Can you work these out from the model? Positions are in its coordinate system, mm. Face numbers are marked on the shaded views. A direction names the side the tool comes from. Round coordinates to 2 decimals unless told otherwise and drop trailing zeros. Write each loop counter-clockwise with the first axis right and the second up, starting at its lowest first coordinate (ties: lowest second). Pieces come first, ordered by that corner, then holes. Notation, with made-up numbers: (-17, 76) -> (32, 76) arc R14 ccw to (32, 80) -> close; hole circle Ø3 at (46, 10). An arc over 180 degrees is marked (long way). Write item = value, one per line. Start each with the question number.
1) If I drill on line 1 (Y direction, x = 154.5, z = 96); line 2 (X direction, y = 126, z = 8); line 3 (Y direction, x = 157.5, z = -145), over which ranges is the centre line in solid material (lowest first)?
2) For the marked faces 1 and 2, which set-ups out of +Z, -Z, +X, -X, +Y, -Y let a thin tool reach every point of the face, with its end or its side?
3) I'm going to push flat-ended pins straight in: pin 1 (24 mm diameter, centred on x = 241, y = 206, fed in from +Z); pin 2 (8 mm diameter, centred on y = 297.5, z = 144, fed in from +X); pin 3 (5.5 mm diameter, centred on x = -153, y = -194.5, fed in from +Z). Where does each tip first touch, or does it pass through?
4) Imagine slicing it at A-A, the plane y = 260.5. Please give me the cut outline in (x, z), then the cut area to 3 significant figures.
5) Imagine slicing it at C-C, the plane x = 54.5. Please give me the cut outline in (y, z).
6) Imagine slicing it at B-B, the plane z = -93.5. State how many separate pieces and enclosed holes the cut face has, then the cut area to 3 significant figures.
7) Imagine slicing it at D-D, the plane x = 182. Please give me the cut outline in (y, z).
8) Thinking about a two-plate mould opening in Y: for the marked faces 3, 4, 5 and 6, which applies, +Y half, -Y half, draft (parallel to the pull), parting line (faces both ways), or undercut?
from build123d import *

# Parameters (mm, degrees)
SKETCH1_W            = 450
SKETCH1_H            = 900
BOSS_EXTRUDE1_DEPTH  = 225
SKETCH2_W            = 390
SKETCH2_H            = 870
CUT_EXTRUDE1_DEPTH   = 420
SKETCH3_W            = 390
SKETCH3_H            = 390
BOSS_EXTRUDE2_DEPTH  = 30
LPATTERN1_COUNT      = 3
LPATTERN1_PITCH      = 155
SKETCH5_W            = 325
SKETCH5_H            = 350.459165748
SKETCH5_W_2          = 265
SKETCH5_H_2          = 290.459165748
BOSS_EXTRUDE4_DEPTH  = 390
SKETCH6_W            = 390
SKETCH6_H            = 125
BOSS_EXTRUDE5_DEPTH  = 10
LPATTERN2_COUNT      = 2
LPATTERN2_PITCH      = 155
LPATTERN2_COUNT_DIR2 = 2
LPATTERN2_PITCH_DIR2 = 320
CUT_EXTRUDE2_REACH   = 632.496
SKETCH10_R           = 2.5
LPATTERN3_COUNT      = 2
LPATTERN3_PITCH      = 155
LPATTERN3_COUNT_DIR2 = 2
LPATTERN3_PITCH_DIR2 = 320
SKETCH13_W           = 450
SKETCH13_H           = 30
BOSS_EXTRUDE6_DEPTH  = 30
CUT_EXTRUDE4_REACH   = 677
SKETCH12_R           = 2.5
CUT_EXTRUDE5_START   = -10
SKETCH17_R           = 2.5
CUT_EXTRUDE5_DEPTH   = 677.276969435
SKETCH18_W           = 53
SKETCH18_H           = 30
CUT_EXTRUDE6_DEPTH   = 676
SKETCH19_W           = 53
SKETCH19_H           = 30
CUT_EXTRUDE7_DEPTH   = 30
SKETCH20_R           = 2.5
CUT_EXTRUDE8_DEPTH   = 10


with BuildPart() as part:
    # Sketch1 → Boss-Extrude1 (new, symmetric)
    with BuildSketch(Plane(origin=(0, 0, 0), x_dir=(0, 0, -1), z_dir=(1, 0, 0))):
        Rectangle(SKETCH1_W, SKETCH1_H)
    extrude(amount=BOSS_EXTRUDE1_DEPTH, both=True)

    # Sketch2 → Cut-Extrude1 (cut)
    with BuildSketch(Plane.XY.offset(225)):
        with Locations((0, -15)):
            Rectangle(SKETCH2_W, SKETCH2_H)
    extrude(amount=-CUT_EXTRUDE1_DEPTH, mode=Mode.SUBTRACT)

    # Sketch3 → Boss-Extrude2 (add)
    with BuildSketch(Plane(origin=(0, 320, 0), x_dir=(1, 0, 0), z_dir=(0, 1, 0))):
        Rectangle(SKETCH3_W, SKETCH3_H)
    boss_extrude2 = extrude(amount=-BOSS_EXTRUDE2_DEPTH)

    # LPattern1: Boss-Extrude2 ×3
    with Locations(*[(0, -i * LPATTERN1_PITCH, 0) for i in range(1, LPATTERN1_COUNT)]):
        add(boss_extrude2)

    # Sketch5 → Boss-Extrude4 (add)
    with BuildSketch(Plane.XY.offset(-195)):
        with Locations((2.5, -274.770417126)):
            Rectangle(SKETCH5_W, SKETCH5_H)
        with Locations((2.5, -274.770417126)):
            Rectangle(SKETCH5_W_2, SKETCH5_H_2, mode=Mode.SUBTRACT)
    extrude(amount=BOSS_EXTRUDE4_DEPTH)

    # Sketch6 → Boss-Extrude5 (add)
    with BuildSketch(Plane(origin=(-165, 0, 0), x_dir=(0, 0, -1), z_dir=(1, 0, 0))):
        with Locations((0, 227.5)):
            Rectangle(SKETCH6_W, SKETCH6_H)
    boss_extrude5 = extrude(amount=BOSS_EXTRUDE5_DEPTH)

    # LPattern2: Boss-Extrude5 2 × 2
    with Locations(*[(j * LPATTERN2_PITCH_DIR2, -i * LPATTERN2_PITCH, 0) for i in range(LPATTERN2_COUNT) for j in range(LPATTERN2_COUNT_DIR2) if (i, j) != (0, 0)]):
        add(boss_extrude5)

    # Sketch10 → Cut-Extrude2 (cut, up to next)
    with BuildSketch(Plane(origin=(-155, 0, 0), x_dir=(0, 0, -1), z_dir=(1, 0, 0)), mode=Mode.PRIVATE) as cut_extrude2_sk1:
        with Locations((-165, 225)):
            Circle(SKETCH10_R)
    cut_extrude2_tool1 = extrude(cut_extrude2_sk1.sketch, amount=-CUT_EXTRUDE2_REACH, mode=Mode.PRIVATE) & part.part
    # Sketch10 → Cut-Extrude2 (cut, up to next)
    with BuildSketch(Plane(origin=(-155, 0, 0), x_dir=(0, 0, -1), z_dir=(1, 0, 0)), mode=Mode.PRIVATE) as cut_extrude2_sk2:
        with Locations((-145, 225)):
            Circle(SKETCH10_R)
    cut_extrude2_tool2 = extrude(cut_extrude2_sk2.sketch, amount=-CUT_EXTRUDE2_REACH, mode=Mode.PRIVATE) & part.part
    # Sketch10 → Cut-Extrude2 (cut, up to next)
    with BuildSketch(Plane(origin=(-155, 0, 0), x_dir=(0, 0, -1), z_dir=(1, 0, 0)), mode=Mode.PRIVATE) as cut_extrude2_sk3:
        with Locations(Location((145, 225, 0), (0, 0, 180))):
            Circle(SKETCH10_R)
    cut_extrude2_tool3 = extrude(cut_extrude2_sk3.sketch, amount=-CUT_EXTRUDE2_REACH, mode=Mode.PRIVATE) & part.part
    # Sketch10 → Cut-Extrude2 (cut, up to next)
    with BuildSketch(Plane(origin=(-155, 0, 0), x_dir=(0, 0, -1), z_dir=(1, 0, 0)), mode=Mode.PRIVATE) as cut_extrude2_sk4:
        with Locations(Location((165, 225, 0), (0, 0, 180))):
            Circle(SKETCH10_R)
    cut_extrude2_tool4 = extrude(cut_extrude2_sk4.sketch, amount=-CUT_EXTRUDE2_REACH, mode=Mode.PRIVATE) & part.part
    cut_extrude2_1 = cut_extrude2_tool1.solids().sort_by_distance((-155, 225, 165))[0]
    add(cut_extrude2_1, mode=Mode.SUBTRACT)
    cut_extrude2_2 = cut_extrude2_tool2.solids().sort_by_distance((-155, 225, 145))[0]
    add(cut_extrude2_2, mode=Mode.SUBTRACT)
    cut_extrude2_3 = cut_extrude2_tool3.solids().sort_by_distance((-155, 225, -145))[0]
    add(cut_extrude2_3, mode=Mode.SUBTRACT)
    cut_extrude2_4 = cut_extrude2_tool4.solids().sort_by_distance((-155, 225, -165))[0]
    add(cut_extrude2_4, mode=Mode.SUBTRACT)
    cut_extrude2 = cut_extrude2_1 + cut_extrude2_2 + cut_extrude2_3 + cut_extrude2_4  # Cut-Extrude2 as one shape, for the pattern or mirror that repeats it

    # LPattern3: Cut-Extrude2 2 × 2
    with Locations(*[(j * LPATTERN3_PITCH_DIR2, -i * LPATTERN3_PITCH, 0) for i in range(LPATTERN3_COUNT) for j in range(LPATTERN3_COUNT_DIR2) if (i, j) != (0, 0)]):
        add(cut_extrude2, mode=Mode.SUBTRACT)

    # Sketch13 → Boss-Extrude6 (add)
    with BuildSketch(Plane(origin=(225, 0, 0), x_dir=(0, 0, -1), z_dir=(1, 0, 0))):
        with Locations((0, 210.86)):
            Rectangle(SKETCH13_W, SKETCH13_H)
    extrude(amount=BOSS_EXTRUDE6_DEPTH)

    # Sketch12 → Cut-Extrude4 (cut, up to next)
    with BuildSketch(Plane(origin=(225, 0, 0), x_dir=(0, 0, -1), z_dir=(1, 0, 0)), mode=Mode.PRIVATE) as cut_extrude4_sk1:
        with Locations(Location((-150, 218.36, 0), (0, 0, 180))):
            Circle(SKETCH12_R)
    cut_extrude4_tool1 = extrude(cut_extrude4_sk1.sketch, amount=CUT_EXTRUDE4_REACH, mode=Mode.PRIVATE) & part.part
    # Sketch12 → Cut-Extrude4 (cut, up to next)
    with BuildSketch(Plane(origin=(225, 0, 0), x_dir=(0, 0, -1), z_dir=(1, 0, 0)), mode=Mode.PRIVATE) as cut_extrude4_sk2:
        with Locations(Location((-110, 218.36, 0), (0, 0, 180))):
            Circle(SKETCH12_R)
    cut_extrude4_tool2 = extrude(cut_extrude4_sk2.sketch, amount=CUT_EXTRUDE4_REACH, mode=Mode.PRIVATE) & part.part
    # Sketch12 → Cut-Extrude4 (cut, up to next)
    with BuildSketch(Plane(origin=(225, 0, 0), x_dir=(0, 0, -1), z_dir=(1, 0, 0)), mode=Mode.PRIVATE) as cut_extrude4_sk3:
        with Locations(Location((-130, 203.36, 0), (0, 0, 180))):
            Circle(SKETCH12_R)
    cut_extrude4_tool3 = extrude(cut_extrude4_sk3.sketch, amount=CUT_EXTRUDE4_REACH, mode=Mode.PRIVATE) & part.part
    # Sketch12 → Cut-Extrude4 (cut, up to next)
    with BuildSketch(Plane(origin=(225, 0, 0), x_dir=(0, 0, -1), z_dir=(1, 0, 0)), mode=Mode.PRIVATE) as cut_extrude4_sk4:
        with Locations(Location((110, 218.36, 0), (0, 0, 180))):
            Circle(SKETCH12_R)
    cut_extrude4_tool4 = extrude(cut_extrude4_sk4.sketch, amount=CUT_EXTRUDE4_REACH, mode=Mode.PRIVATE) & part.part
    # Sketch12 → Cut-Extrude4 (cut, up to next)
    with BuildSketch(Plane(origin=(225, 0, 0), x_dir=(0, 0, -1), z_dir=(1, 0, 0)), mode=Mode.PRIVATE) as cut_extrude4_sk5:
        with Locations(Location((130, 203.36, 0), (0, 0, 180))):
            Circle(SKETCH12_R)
    cut_extrude4_tool5 = extrude(cut_extrude4_sk5.sketch, amount=CUT_EXTRUDE4_REACH, mode=Mode.PRIVATE) & part.part
    # Sketch12 → Cut-Extrude4 (cut, up to next)
    with BuildSketch(Plane(origin=(225, 0, 0), x_dir=(0, 0, -1), z_dir=(1, 0, 0)), mode=Mode.PRIVATE) as cut_extrude4_sk6:
        with Locations(Location((150, 218.36, 0), (0, 0, 180))):
            Circle(SKETCH12_R)
    cut_extrude4_tool6 = extrude(cut_extrude4_sk6.sketch, amount=CUT_EXTRUDE4_REACH, mode=Mode.PRIVATE) & part.part
    add(cut_extrude4_tool1.solids().sort_by_distance((225, 218.36, 150))[0], mode=Mode.SUBTRACT)
    add(cut_extrude4_tool2.solids().sort_by_distance((225, 218.36, 110))[0], mode=Mode.SUBTRACT)
    add(cut_extrude4_tool3.solids().sort_by_distance((225, 203.36, 130))[0], mode=Mode.SUBTRACT)
    add(cut_extrude4_tool4.solids().sort_by_distance((225, 218.36, -110))[0], mode=Mode.SUBTRACT)
    add(cut_extrude4_tool5.solids().sort_by_distance((225, 203.36, -130))[0], mode=Mode.SUBTRACT)
    add(cut_extrude4_tool6.solids().sort_by_distance((225, 218.36, -150))[0], mode=Mode.SUBTRACT)

    # Sketch17 → Cut-Extrude5 (cut)
    with BuildSketch(Plane.XY.offset(195).offset(CUT_EXTRUDE5_START)):
        with Locations(Location((-152.5, -194.540834252, 0), (0, 0, 180))):
            Circle(SKETCH17_R)
        with Locations(Location((-137.5, -174.540834252, 0), (0, 0, 180))):
            Circle(SKETCH17_R)
        with Locations(Location((-152.5, -154.540834252, 0), (0, 0, 180))):
            Circle(SKETCH17_R)
    cut_extrude5 = extrude(amount=CUT_EXTRUDE5_DEPTH, mode=Mode.SUBTRACT)

    # Mirror1: Cut-Extrude5 across plane
    add(cut_extrude5.mirror(Plane.ZX.offset(-269.770834252)), mode=Mode.SUBTRACT)

    # Sketch18 → Cut-Extrude6 (cut, through all)
    with BuildSketch(Plane(origin=(225, 0, 0), x_dir=(0, 0, -1), z_dir=(1, 0, 0))):
        with Locations((-198.5, 210.86)):
            Rectangle(SKETCH18_W, SKETCH18_H)
    extrude(amount=CUT_EXTRUDE6_DEPTH, mode=Mode.SUBTRACT)

    # Sketch19 → Cut-Extrude7 (cut)
    with BuildSketch(Plane(origin=(255, 0, 0), x_dir=(0, 0, -1), z_dir=(1, 0, 0))):
        with Locations((198.5, 210.86)):
            Rectangle(SKETCH19_W, SKETCH19_H)
    extrude(amount=-CUT_EXTRUDE7_DEPTH, mode=Mode.SUBTRACT)

    # Sketch20 → Cut-Extrude8 (cut)
    with BuildSketch(Plane(origin=(255, 0, 0), x_dir=(0, 0, -1), z_dir=(1, 0, 0))):
        with Locations((-20, 218.36)):
            Circle(SKETCH20_R)
        with Locations((0, 203.36)):
            Circle(SKETCH20_R)
        with Locations((20, 218.36)):
            Circle(SKETCH20_R)
    extrude(amount=-CUT_EXTRUDE8_DEPTH, mode=Mode.SUBTRACT)


solid = part.part
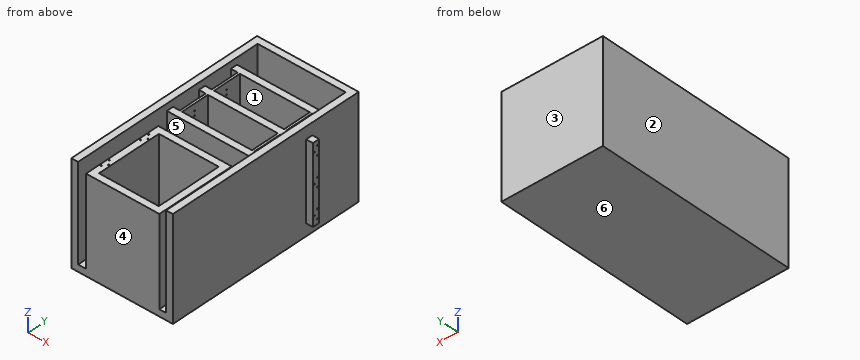
Reported:
q1.line_1 = -450 to -99.54, -20 to 10, 135 to 165, 290 to 320, 420 to 450
q1.line_2 = -225 to -195, -165 to -155, 155 to 165, 195 to 225
q1.line_3 = -450 to -99.54, -20 to 67.5, 72.5 to 222.5, 227.5 to 320, 420 to 450
q2.face_1 = +Z
q2.face_2 = +Z, -Z, -X, +Y, -Y
q3.pin_1 = 172
q3.pin_2 = 225
q3.pin_3 = 195
q4.outline = (-225, -225) -> (225, -225) -> (225, 225) -> (195, 225) -> (195, -195) -> (165, -195) -> (165, 195) -> (155, 195) -> (155, -195) -> (-155, -195) -> (-155, 195) -> (-165, 195) -> (-165, -195) -> (-195, -195) -> (-195, 225) -> (-225, 225) -> close
q4.area = 46,500 mm²
q5.outline = (-450, -225) -> (450, -225) -> (450, 225) -> (420, 225) -> (420, -195) -> (320, -195) -> (320, 195) -> (290, 195) -> (290, -195) -> (165, -195) -> (165, 195) -> (135, 195) -> (135, -195) -> (10, -195) -> (10, 195) -> (-20, 195) -> (-20, -195) -> (-99.54, -195) -> (-99.54, 195) -> (-129.54, 195) -> (-129.54, -195) -> (-420, -195) -> (-420, 195) -> (-450, 195) -> close
q6.separate_pieces = 2
q6.enclosed_holes = 8
q6.area = 144,000 mm²
q7.outline = (-450, -225) -> (450, -225) -> (450, 225) -> (420, 225) -> (420, -195) -> (320, -195) -> (320, 195) -> (290, 195) -> (290, -195) -> (165, -195) -> (165, 195) -> (135, 195) -> (135, -195) -> (10, -195) -> (10, 195) -> (-20, 195) -> (-20, -195) -> (-450, -195) -> close
q8.face_3 = +Y half
q8.face_4 = -Y half
q8.face_5 = undercut
q8.face_6 = draft
